Could you check a few things on this model? Use its own coordinates, in mm. Give positions to 0.01 mm unless a question says otherwise; leave off trailing zeros. Loops run counter-clockwise (first coordinate to the right, second up) from the corner with the lowest first, then second, coordinate; pieces in that order, holes last. Notation, with made-up numbers: (6, 19) -> (11, 19) arc R16 ccw to (11, 43) -> close; hole circle Ø11 at (-38.5, -38). An arc over 180 degrees is marked (long way). Put each result on its own line as item: value.
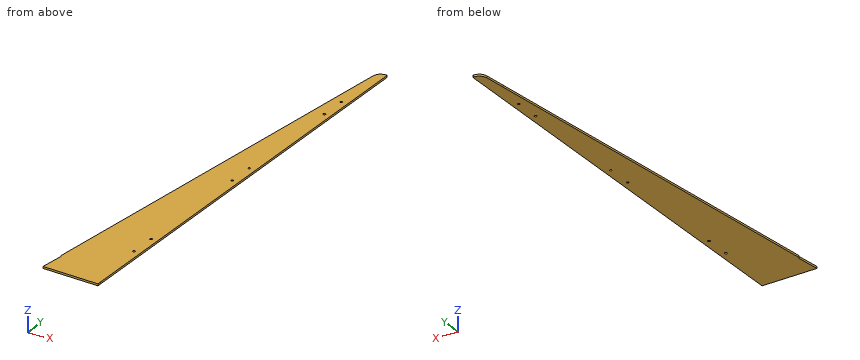
```python
from build123d import *

# Parameters (mm, degrees)
BOSS_EXTRUDE1_DEPTH = 5
FILLET1_R           = 2
BOSS_EXTRUDE2_DEPTH = 5
BOSS_EXTRUDE3_DEPTH = 5
BOSS_EXTRUDE4_DEPTH = 5
CUT_EXTRUDE1_DEPTH  = 1184.176367894
SKETCH6_R           = 3.25
CUT_EXTRUDE2_DEPTH  = 1184.176367894
BOSS_EXTRUDE5_DEPTH = 5
CUT_EXTRUDE3_DEPTH  = 1184.176367894
SKETCH9_R           = 3
CUT_EXTRUDE4_DEPTH  = 1184.176367894


with BuildPart() as part:
    # Sketch1 → Boss-Extrude1 (new body)
    with BuildSketch(Plane.XY):
        Polygon((0, 0), (148, 0), (210.710741947, 1195), align=None)
    extrude(amount=BOSS_EXTRUDE1_DEPTH)

    # Fillet1
    fillet1_edges = [part.edges().sort_by_distance(p)[0] for p in [
        (210.710741947, 1195, 2.5),
    ]]
    fillet(fillet1_edges, radius=FILLET1_R)

    # Sketch2 → Boss-Extrude2 (add)
    with BuildSketch(Plane.XY.offset(5)):
        Polygon((191.942300905, 1088.558881537), (174.215761351, 1091.684548735), (10.318366476, 72.915290412), (12.780385859, 72.481169967), align=None)
    extrude(amount=-BOSS_EXTRUDE2_DEPTH)

    # Sketch3 → Boss-Extrude3 (add)
    with BuildSketch(Plane.XY.offset(5)):
        with BuildLine():
            Line((174.215761351, 1091.684548735), (182.955612005, 1146.010556635))
            ThreePointArc((182.955612005, 1146.010556635), (191.401570157, 1160.078122114), (207.225341391, 1164.418499006))
            ThreePointArc((207.225341391, 1164.418499006), (205.802244472, 1164.033891637), (205.029250268, 1162.778659534))
            Line((205.029250268, 1162.778659534), (191.942300905, 1088.558881537))
            Line((191.942300905, 1088.558881537), (174.215761351, 1091.684548735))
        make_face()
    extrude(amount=-BOSS_EXTRUDE3_DEPTH)

    # Sketch4 → Boss-Extrude4 (add)
    with BuildSketch(Plane.XY.offset(5)):
        Polygon((0, 0), (2.112629849, 11.981319257), (148.088309576, 1.682804887), (148, 0), align=None)
    extrude(amount=-BOSS_EXTRUDE4_DEPTH)

    # Sketch5 → Cut-Extrude1 (cut, through all)
    with BuildSketch(Plane.XY.offset(5)):
        Polygon((148.679280264, 12.9441925), (0.545384836, 3.093031107), (0, 0), (148, 0), align=None)
    extrude(amount=-CUT_EXTRUDE1_DEPTH, mode=Mode.SUBTRACT)

    # Sketch6 → Cut-Extrude2 (cut, through all)
    with BuildSketch(Plane.XY.offset(5)):
        with Locations((180.368599434, 937.514146328)):
            Circle(SKETCH6_R)
        with Locations((183.932173312, 1005.420706697)):
            Circle(SKETCH6_R)
        with Locations((143.832770259, 241.296648182)):
            Circle(SKETCH6_R)
        with Locations((140.269196381, 173.390087812)):
            Circle(SKETCH6_R)
    extrude(amount=-CUT_EXTRUDE2_DEPTH, mode=Mode.SUBTRACT)

    # Sketch7 → Boss-Extrude5 (add)
    with BuildSketch(Plane.XY.offset(5)):
        Polygon((148.679280264, 12.9441925), (148.090399515, 1.722630236), (54.104333141, 6.654794215), align=None)
    extrude(amount=-BOSS_EXTRUDE5_DEPTH)

    # Sketch8 → Cut-Extrude3 (cut, through all)
    with BuildSketch(Plane.XY.offset(5)):
        Polygon((54.104333141, 6.654794215), (1.658710562, 9.407015055), (0.545384836, 3.093031107), align=None)
    extrude(amount=-CUT_EXTRUDE3_DEPTH, mode=Mode.SUBTRACT)

    # Sketch9 → Cut-Extrude4 (cut, through all)
    with BuildSketch(Plane.XY.offset(5)):
        with Locations((160.968231329, 567.825650117)):
            Circle(SKETCH9_R)
        with Locations((164.531805206, 635.732210487)):
            Circle(SKETCH9_R)
    extrude(amount=-CUT_EXTRUDE4_DEPTH, mode=Mode.SUBTRACT)


solid = part.part
```
1. I need wall thicknesses on line 1 (X direction, y = 961, z = 3.2); line 2 (X direction, y = 665, z = 4.05). Which ranges of each line are inside material? Lowest first, please.
Recorded:
line 1: x = 153.19 to 198.43
line 2: x = 105.57 to 182.9
2. If we section it at B-B (y = 94.5): List the corners of the cut face in (x, z) for me, then the cut area to 3 significant figures.
Recorded:
outline: (13.79, 0) -> (152.96, 0) -> (152.96, 5) -> (13.79, 5) -> close
area: 696 mm^2
3. I'm going to push flat-ended pins straight in: pin 1 (2 mm diameter, centred on x = 82.5, z = 3, fed in from -Y); pin 2 (2 mm diameter, centred on y = 249, z = 4, fed in from +X); pin 3 (2 mm diameter, centred on y = 879, z = 1.5, fed in from -X). Where does each tip first touch, or does it pass through?
Recorded:
pin 1: stops at y = 5.11
pin 2: stops at x = 161.12
pin 3: stops at x = 139.84
4. If we section it at C-C (x = 52): List the corners of the cut face in (y, z) for me.
Recorded:
outline: (6.77, 0) -> (332, 0) -> (332, 5) -> (6.77, 5) -> close
5. If we section it at A-A (z = 1.7): List the corners of the cut face in (x, y) for me, then the cut area to 3 significant figures.
Recorded:
outline: (1.66, 9.41) -> (148.09, 1.72) -> (209, 1162.33) arc R2 ccw to (207.23, 1164.42) arc R22.05 ccw to (182.96, 1146.01) -> (10.32, 72.92) -> (12.78, 72.48) -> close; hole circle Ø6.5 at (140.27, 173.39); hole circle Ø6.5 at (143.83, 241.3); hole circle Ø6 at (160.97, 567.83); hole circle Ø6 at (164.53, 635.73); hole circle Ø6.5 at (180.37, 937.51); hole circle Ø6.5 at (183.93, 1005.42)
area: 99,300 mm^2
